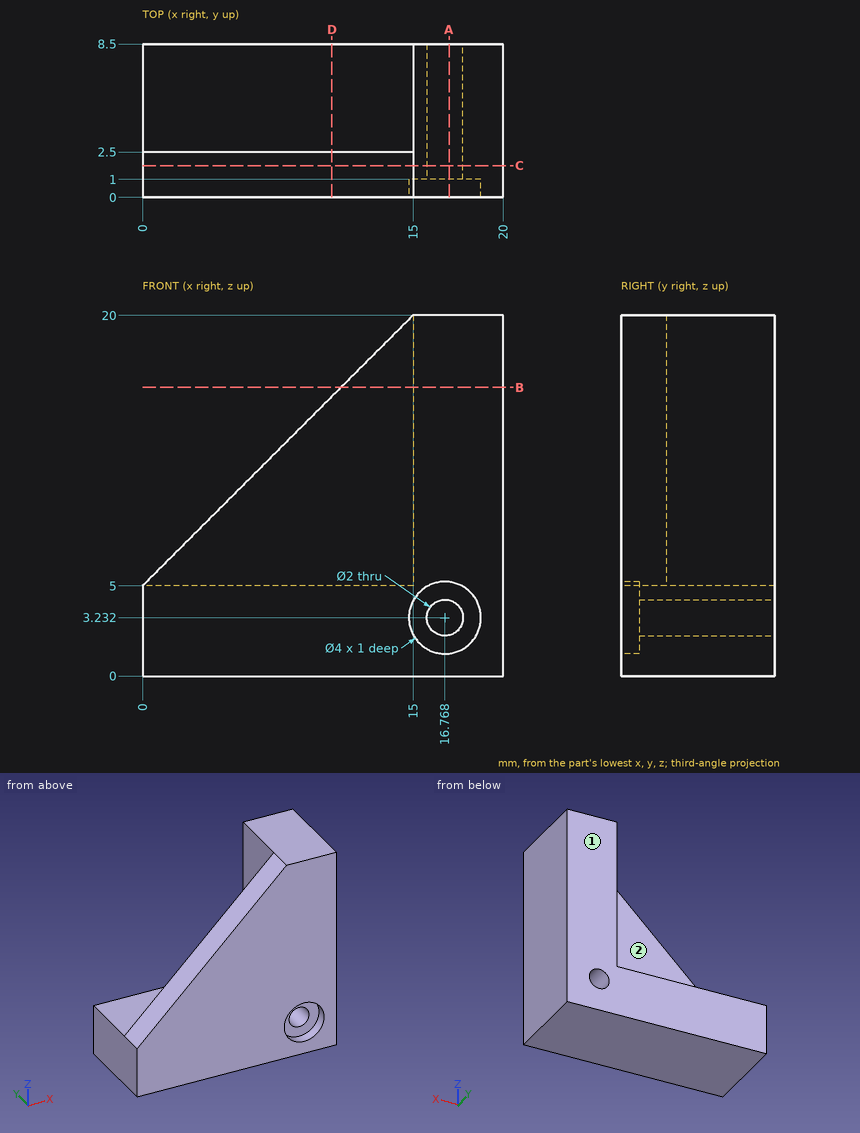
Source: three-view drawing plus pictorial views. Frame: mm from the lowest corner of the part. A direction names the side the tool comes from. Give positions to 0.01 mm unless a question says otherwise; leave off trailing zeros. Order: outer loops, then holes, each group sorted by start corner. A loop starts at its lowest first (then second) coordinate and runs counter-clockwise, first axis right, second up. Notation, with made-up numbers: (-33, 15.5) -> (-3, 15.5) arc R19 cw to (-3, 32.5) -> close; hole circle Ø7 at (60, 72.5). An arc over 180 degrees is marked (long way). Write each question's results on one line, items separated by ' | '. Start each with the question number.
Item 1: Set-up query: the marked faces 1 and 2. Return all of +Z, -Z, +X, -X, +Y, -Y with unobstructed straight access to the full face (end or side cutting, diameter ignored); none if empty.
Item 2: Cut plane B-B on z = 16. Return the cut outline in (x, y), then the cut area to 3 significant figures.
Item 3: Line query: line 1 (X direction, y = 7, z = 6.25); line 2 (Y direction, x = 14.25, z = 14.5); line 3 (Z direction, x = 6.25, y = 5). Output: solid intervals per line, ascending.
Item 4: Cut plane C-C on y = 1.75. Return the cut outline in (x, z).
Item 5: Contact query for flat-ended pins moving along their axis: P1, Ø2.5, axis at x = 16.77, z = 3.23, coming from the -Y side; P2, Ø3, axis at x = 4, y = 5.5, coming from the +Z side; P3, Ø1.8, axis at y = 5.5, z = 11.5, coming from the -X side. Output: stop coordinate, or through.
Item 6: Cut plane A-A on x = 17. Return the cut outline in (y, z) (1 decimal), then the cut area to 3 significant figures.
Item 7: Cut plane D-D on x = 10.5. Return the cut outline in (y, z).
Established:
1) face 1: +Z, -Z, +X, -X, +Y | face 2: +Z, -X, +Y
2) outline: (11, 0) -> (20, 0) -> (20, 8.5) -> (15, 8.5) -> (15, 2.5) -> (11, 2.5) -> close | area: 52.5 mm^2
3) line 1: 15 to 20 | line 2: 0 to 2.5 | line 3: 0 to 5
4) outline: (0, 0) -> (20, 0) -> (20, 20) -> (15, 20) -> (0, 5) -> close; hole circle Ø2 at (16.77, 3.23)
5) P1: y = 1 | P2: z = 5 | P3: x = 15
6) outline: (0, 0) -> (8.5, 0) -> (8.5, 2.3) -> (1, 2.3) -> (1, 1.2) -> (0, 1.2) -> close; (0, 5.2) -> (1, 5.2) -> (1, 4.2) -> (8.5, 4.2) -> (8.5, 20) -> (0, 20) -> close | area: 151 mm^2
7) outline: (0, 0) -> (8.5, 0) -> (8.5, 5) -> (2.5, 5) -> (2.5, 15.5) -> (0, 15.5) -> close
